```python
from build123d import *

# Parameters (mm, degrees)
BOSS_EXTRUDE1_DEPTH                                  = 7
CUT_EXTRUDE1_DEPTH                                   = 4
CSK_FOR_M3_HEX_SOCKET_COUNTERSUNK_CAP_SC_D           = 3.4
CSK_FOR_M3_HEX_SOCKET_COUNTERSUNK_CAP_SC_DEPTH       = 7.5
CSK_FOR_M3_HEX_SOCKET_COUNTERSUNK_CAP_SC_CSINK_D     = 6.72
CSK_FOR_M3_HEX_SOCKET_COUNTERSUNK_CAP_SC_CSINK_ANGLE = 90
CSK_FOR_M3_HEX_SOCKET_COUNTERSUNK_CAP_SC_TIP         = 1.021463052
HOLE1_D                                              = 4.15
CUT_EXTRUDE2_DEPTH                                   = 4
CHAMFER1_SIZE                                        = 0.5


with BuildPart() as part:
    # Sketch1 → Boss-Extrude1 (new body)
    with BuildSketch(Plane(origin=(0, 0, 0), x_dir=(1, 0, 0), z_dir=(0, 1, 0))):
        with BuildLine():
            Line((0, 5), (8.5, 5))
            ThreePointArc((8.5, 5), (13.5, 0), (8.5, -5))
            Line((8.5, -5), (0, -5))
            ThreePointArc((0, -5), (-5, 0), (0, 5))
        make_face()
    extrude(amount=BOSS_EXTRUDE1_DEPTH)

    # Sketch2 → Cut-Extrude1 (cut)
    with BuildSketch(Plane(origin=(0, 7, 0), x_dir=(1, 0, 0), z_dir=(0, 1, 0))):
        with BuildLine():
            ThreePointArc((-1.5, 2), (-2.5, 0), (-1.5, -2))
            Line((-1.5, -2), (1.5, -2))
            ThreePointArc((1.5, -2), (2.236067977, -1.118033989), (2.5, 0))
            ThreePointArc((2.5, 0), (2.236067977, 1.118033989), (1.5, 2))
            Line((1.5, 2), (-1.5, 2))
        make_face()
    extrude(amount=-CUT_EXTRUDE1_DEPTH, mode=Mode.SUBTRACT)

    # CSK for M3 Hex Socket Countersunk Cap Screw2
    with Locations(Plane(origin=(0, 0, 0), x_dir=(-1, 0, 0), z_dir=(0, -1, 0))):
        with Locations((0, 0)):
            CounterSinkHole(CSK_FOR_M3_HEX_SOCKET_COUNTERSUNK_CAP_SC_D / 2, CSK_FOR_M3_HEX_SOCKET_COUNTERSUNK_CAP_SC_CSINK_D / 2, depth=CSK_FOR_M3_HEX_SOCKET_COUNTERSUNK_CAP_SC_DEPTH, counter_sink_angle=CSK_FOR_M3_HEX_SOCKET_COUNTERSUNK_CAP_SC_CSINK_ANGLE)
            with Locations((0, 0, -(CSK_FOR_M3_HEX_SOCKET_COUNTERSUNK_CAP_SC_DEPTH + CSK_FOR_M3_HEX_SOCKET_COUNTERSUNK_CAP_SC_TIP / 2))):  # 118° drill point
                Cone(0, CSK_FOR_M3_HEX_SOCKET_COUNTERSUNK_CAP_SC_D / 2, CSK_FOR_M3_HEX_SOCKET_COUNTERSUNK_CAP_SC_TIP, mode=Mode.SUBTRACT)

    # Hole1 (through all)
    with Locations(Plane(origin=(0, 0, 0), x_dir=(-1, 0, 0), z_dir=(0, -1, 0))):
        with Locations((-8.5, 0)):
            Hole(HOLE1_D / 2)

    # Sketch11 → Cut-Extrude2 (cut)
    with BuildSketch(Plane(origin=(0, 7, 0), x_dir=(1, 0, 0), z_dir=(0, 1, 0))):
        Polygon((11.848631561, 0), (10.174315781, 2.9), (6.825684219, 2.9), (5.151368439, 0), (6.825684219, -2.9), (10.174315781, -2.9), align=None)
    extrude(amount=-CUT_EXTRUDE2_DEPTH, mode=Mode.SUBTRACT)

    # Chamfer1
    chamfer1_edges = [part.edges().sort_by_distance(p)[0] for p in [
        (13.5, 7, 0),
        (0, 7, -2),
        (4.25, 7, -5),
        (-2.5, 7, 0),
        (0, 7, 2),
        (2.5, 7, 0),
        (-5, 7, 0),
        (4.25, 0, -5),
        (13.5, 0, 0),
        (4.25, 0, 5),
        (-5, 0, 0),
        (4.25, 7, 5),
    ]]
    chamfer(chamfer1_edges, length=CHAMFER1_SIZE)


solid = part.part
```
Work out the finished part from the listing and answer in its coordinate system (mm). A direction names the side the tool comes from. Give positions to 0.01 mm unless a question says otherwise; leave off trailing zeros. Loops run counter-clockwise (first coordinate to the right, second up) from the corner with the lowest first, then second, coordinate; pieces in that order, holes last. Notation, with made-up numbers: (0, -23.5) - (43, -23.5) arc R23 cw to (43, -10.5) - close; hole circle Ø7 at (-37, 79). An arc over 180 degrees is marked (long way). Use CSV: the item, a comma, the result in double quotes. Start each with the question number.
(1) Find the intervals of material crossed by L1, parallel to Z at x = 8.5, y = 0.65 (3 decimals); L2, parallel to X at y = 5.5, z = -1.25; L3, parallel to Z at x = 0, y = 2.45, in increasing order.
(2) Find section C-C, the plane z = 1.5. Count the separate pieces of the cut face and the enclosed holes in it, plus the area to 3 significant figures.
(3) Each of these flat-tipped pins is pushed along its axis until it touches: pin 1 (1 mm diameter, centred on x = -2, z = -3, fed in from -Y); pin 2 (2 mm diameter, centred on x = 10.5, y = 1, fed in from -Z); pin 3 (1 mm diameter, centred on y = 6.5, z = 4, fed in from +X). Where does it stop, or does it pass through?
(4) Find section B-B, the plane x = 5.75. Determine the outline of the cut face in (y, z).
(5) A tool of negligible diameter and unlimited length cuts with its end or side. For faces 4 (the face through (11, 5.03, 1.47)), 5 (the face through (13.5, 3.5, -0.1)), from which of +Z, -Z, +X, -X, +Y, -Y can it reach the whole face along a straight path? Write none if from no direction.
(6) Find section A-A, the plane y = 6. Determine the outline of the cut face in (x, z), plus the area to 3 significant figures.
(7) Determine the mould class of faces 1 (the face through (13.134, 6.865, -0.102)), 2 (the face through (5.977, 5.028, 1.43)), 3 (the face through (-4.634, 6.865, 0.102)) for opening direction X: released by +X, released by -X, zero draft, split by the parting line, or undercut.
(8) Find section D-D, the plane y = 1.25. Determine the outline of the cut face in (x, z) (3 decimals).
Results found:
1,L1,"-5 to -2.075, 2.075 to 5"
1,L2,"-4.84 to -2.17, 2.17 to 5.87, 11.13 to 13.34"
1,L3,"-5 to -1.7, 1.7 to 5"
2,separate pieces,"3"
2,enclosed holes,"0"
2,area,"72.2 mm^2"
3,pin 1,"y = 0"
3,pin 2,"z = -4.9"
3,pin 3,"x = 12.07"
4,outline,"(0, -4.5) - (0.5, -5) - (6.5, -5) - (7, -4.5) - (7, -1.04) - (3, -1.04) - (3, 1.04) - (7, 1.04) - (7, 4.5) - (6.5, 5) - (0.5, 5) - (0, 4.5) - close"
5,face 4,"+Y"
5,face 5,"+X, +Y, -Y"
6,outline,"(0, -5) - (8.5, -5) arc R5 ccw to (8.5, 5) - (0, 5) arc R5 ccw to start; hole (-1.5, -2) - (1.5, -2) arc R2.5 ccw to (1.5, 2) - (-1.5, 2) arc R2.5 ccw to start; hole (5.15, 0) - (6.83, -2.9) - (10.17, -2.9) - (11.85, 0) - (10.17, 2.9) - (6.83, 2.9) - close"
6,area,"117 mm^2"
7,face 1,"released by +X"
7,face 2,"undercut"
7,face 3,"released by -X"
8,outline,"(0, -5) - (8.5, -5) arc R5 ccw to (8.5, 5) - (0, 5) arc R5 ccw to start; hole circle Ø4.22 at (0, 0); hole circle Ø4.15 at (8.5, 0)"
